Here's how the part is built. I have some questions about the finished solid (model axes, mm). A direction names the side the tool comes from. Coordinates: 2 decimals unless noted, no trailing zeros. Loops run counter-clockwise (first coordinate to the right, second up) from the corner with the lowest first, then second, coordinate; pieces in that order, holes last. Notation, with made-up numbers: (2.25, 11.25) - (27.25, 11.25) arc R18 ccw to (27.25, 25.25) - close; hole circle Ø4 at (23, 0). An arc over 180 degrees is marked (long way). Use a Markdown table: item, result.
Autodesk Inventor part; units mm, degrees
ref_plane "YZ Plane" through (0, 0, 0) normal (1, 0, 0) x (0, 1, 0)
ref_plane "XZ Plane" through (0, 0, 0) normal (0, 1, 0) x (-1, 0, 0)
ref_plane "XY Plane" through (0, 0, 0) normal (0, 0, 1) x (1, 0, 0)
sketch "スケッチ1" plane through (0, 0, 0) normal (0, 0, 1) x (1, 0, 0)
  line L0 (-70, 70) -> (70, 70)
  line L1 (70, 70) -> (70, -70)
  line L2 (70, -70) -> (-70, -70)
  line L3 (-70, -70) -> (-70, 70)
  line L4 (-62.5, 62.5) -> (62.5, 62.5) construction
  line L5 (62.5, 62.5) -> (62.5, -62.5) construction
  line L6 (62.5, -62.5) -> (-62.5, -62.5) construction
  line L7 (-62.5, -62.5) -> (-62.5, 62.5) construction
  circle A0 centre (-62.5, 62.5) radius 1.65
  line L8 (-30.5, 62.5) -> (30.5, 62.5)
  line L9 (62.5, 30.5) -> (62.5, -30.5)
  line L10 (30.5, -62.5) -> (-30.5, -62.5)
  line L11 (-62.5, -30.5) -> (-62.5, 30.5)
  arc A1 (-30.5, 62.5) -> (-62.5, 30.5) centre (-30.5, 30.5) ccw
  arc A2 (-62.5, -30.5) -> (-30.5, -62.5) centre (-30.5, -30.5) ccw
  arc A3 (30.5, -62.5) -> (62.5, -30.5) centre (30.5, -30.5) ccw
  arc A4 (62.5, 30.5) -> (30.5, 62.5) centre (30.5, 30.5) ccw
  line L12 (53.1274, 53.1274) -> (-53.1274, -53.1274) construction
  circle A5 centre (-62.5, -62.5) radius 1.65
  circle A6 centre (62.5, -62.5) radius 1.65
  circle A7 centre (62.5, 62.5) radius 1.65
  point P0 (0, 0)
  point P1 (-70, 0)
  point P2 (0, 70)
  point P3 (-62.5, 0)
  point P4 (0, 62.5)
  dimension "d0" = 140
  dimension "d1" = 125
  dimension "d3" = 3.3
  dimension "d4" = 32
  dimension "d5" = 150.267
extrude "押し出し1" add sketch "スケッチ1" along normal blind 4
sketch "スケッチ2" plane through (0, 0, 4) normal (0, 0, 1) x (1, 0, 0)
  line L0 (-70, 70) -> (-70, -70) construction
  line L1 (70, -70) -> (70, 70) construction
  line L2 (-70, 70) -> (-75, 70)
  line L3 (-75, 70) -> (-75, -70)
  line L4 (-75, -70) -> (-70, -70)
  line L5 (-70, -70) -> (-70, 70)
  line L6 (70, 70) -> (75, 70)
  line L7 (75, 70) -> (75, -70)
  line L8 (75, -70) -> (70, -70)
  line L9 (70, -70) -> (70, 70)
  point P0 (0, 0)
  dimension "d8" = 150
extrude "押し出し2" add sketch "スケッチ2" against normal up to surface (4 mm away)
sketch "スケッチ3" plane through (0, 0, 4) normal (0, 0, 1) x (1, 0, 0)
  line L0 (-75, 70) -> (-75, -70) construction
  line L1 (75, 70) -> (75, -70) construction
  line L2 (-75, 70) -> (-70.2, 70)
  line L3 (-70.2, 70) -> (-70.2, -70)
  line L4 (-70.2, -70) -> (-75, -70)
  line L5 (-75, -70) -> (-75, 70)
  line L6 (75, 70) -> (70.2, 70)
  line L7 (70.2, 70) -> (70.2, -70)
  line L8 (70.2, -70) -> (75, -70)
  line L9 (75, -70) -> (75, 70)
  point P0 (0, 0)
  dimension "d11" = 140.4
extrude "押し出し3" add sketch "スケッチ3" along normal blind 4
sketch "スケッチ5" plane through (0, 0, 0) normal (0, 0, -1) x (-1, 0, 0)
  line L0 (75, -70) -> (75, 70) construction
  line L1 (-75, 70) -> (-75, -70) construction
  line L2 (65, -70) -> (65, 70) construction
  line L3 (-65, 70) -> (-65, -70) construction
  circle A0 centre (65, -50) radius 2.25
  circle A1 centre (-65, -50) radius 2.25
  circle A2 centre (65, 50) radius 2.25
  circle A3 centre (-65, 50) radius 2.25
  circle A4 centre (65, -50) radius 7.5 construction
  point P0 (0, 0)
  dimension "d14" = 10
  dimension "d15" = 10
  dimension "d16" = 4.5
  dimension "d17" = 50
  dimension "d18" = 50
  dimension "d19" = 15
extrude "押し出し4" cut sketch "スケッチ5" against normal through all
sketch "スケッチ6" plane through (0, 0, 4) normal (0, 0, 1) x (1, 0, 0)
  circle A0 centre (-65, -50) radius 2.25 construction
  circle A1 centre (65, -50) radius 2.25 construction
  circle A2 centre (65, 50) radius 2.25 construction
  circle A3 centre (-65, 50) radius 2.25 construction
  circle A4 centre (-65, -50) radius 4.25
  circle A5 centre (-65, 50) radius 4.25
  circle A6 centre (65, -50) radius 4.25
  circle A7 centre (65, 50) radius 4.25
  point P0 (0, 0)
  dimension "d22" = 8.5
extrude "押し出し5" cut sketch "スケッチ6" against normal blind 1.5
fillet "フィレット1" radius 2 4 edges at (70.2, 70, 6) (70.2, -70, 6) (-70.2, -70, 6) (-70.2, 70, 6)
properties part number "bottom_140mm_2" material "アルミニウム 6061"
Q1. I want a section at A-A, the plane z = 6. Write out the boundary of the cut face in (x, y).
Check values:
| item | result |
|---|---|
| outline | (-75, -70) - (-72.2, -70) arc R2 ccw to (-70.2, -68) - (-70.2, 68) arc R2 ccw to (-72.2, 70) - (-75, 70) - close; (70.2, -68) arc R2 ccw to (72.2, -70) - (75, -70) - (75, 70) - (72.2, 70) arc R2 ccw to (70.2, 68) - close |
Q2. I want a section at C-C, the plane y = 50. Write out the boundary of the cut face in (x, z).
Check values:
| item | result |
|---|---|
| outline | (-75, 0) - (-67.25, 0) - (-67.25, 2.5) - (-69.25, 2.5) - (-69.25, 4) - (-70.2, 4) - (-70.2, 8) - (-75, 8) - close; (-62.75, 0) - (-55.87, 0) - (-55.87, 4) - (-60.75, 4) - (-60.75, 2.5) - (-62.75, 2.5) - close; (55.87, 0) - (62.75, 0) - (62.75, 2.5) - (60.75, 2.5) - (60.75, 4) - (55.87, 4) - close; (67.25, 0) - (75, 0) - (75, 8) - (70.2, 8) - (70.2, 4) - (69.25, 4) - (69.25, 2.5) - (67.25, 2.5) - close |
Q3. Will these pins go through, and if not, where does the flat tip stop? P1, Ø2.5, axis at x = -64.5, y = 48.5, coming from the +Z side; P2, Ø5.5, axis at x = -62.5, y = -62.5, coming from the +Z side.
Check values:
| item | result |
|---|---|
| P1 | z = 2.5 |
| P2 | z = 4 |
Q4. Please list where these lines run through material, in increasing order: L1, parallel to Y at x = -65, z = 1.05; L2, parallel to Y at x = 65, z = 3.65; L3, parallel to X at y = 20.5, z = 0.5. Write a range as from..to.
Check values:
| item | result |
|---|---|
| L1 | -70..-52.25, -47.75..47.75, 52.25..70 |
| L2 | -70..-54.25, -45.75..45.75, 54.25..70 |
| L3 | -75..-62.5, 62.5..75 |
Q5. I want a section at D-D, the plane x = 32.5. Write out the boundary of the cut face in (y, z), then the cut area to 3 significant figures.
Check values:
| item | result |
|---|---|
| outline | (-70, 0) - (-62.44, 0) - (-62.44, 4) - (-70, 4) - close; (62.44, 0) - (70, 0) - (70, 4) - (62.44, 4) - close |
| area | 60.5 mm^2 |
Q6. I want a section at B-B, the plane y = -1. Write out the boundary of the cut face in (x, z), then the cut area to 3 significant figures.
Check values:
| item | result |
|---|---|
| outline | (-75, 0) - (-62.5, 0) - (-62.5, 4) - (-70.2, 4) - (-70.2, 8) - (-75, 8) - close; (62.5, 0) - (75, 0) - (75, 8) - (70.2, 8) - (70.2, 4) - (62.5, 4) - close |
| area | 138 mm^2 |
Q7. Which directions (+Z, -Z, +X, -X, +Y, -Y) give clear straight access to the entire face, cutting with the end or side of a thin tool? Please do faces 1 (the face through (53.37, -52.88, 1.97)), 2 (the face through (-61.074, -51.628, 3.26)), 3 (the face through (-70.2, 1, 6)).
Check values:
| item | result |
|---|---|
| face 1 | +Z, -Z |
| face 2 | +Z |
| face 3 | +Z, +Y, -Y |
Q8. If we mould it in two halves opening along Y, with no side actions, what happens to faces 4 (the face through (52.88, 53.37, 1.97)), 5 (the face through (70.2, 1, 6)), 6 (the face through (-1, 70, 2))? For each: pulls with the +Y half, pulls with the -Y half, needs draft (parallel to the pull), parting line crosses it, or undercut.
Check values:
| item | result |
|---|---|
| face 4 | undercut |
| face 5 | needs draft |
| face 6 | pulls with the +Y half |
